Study the drawing (mm; zero at the part's minimum x, y, z) and answer. Round coordinates to 2 decimals unless told otherwise and drop trailing zeros. Write each loop counter-clockwise with the first axis right and the second up, starting at its lowest first coordinate (ties: lowest second). Pieces come first, ordered by that corner, then holes.
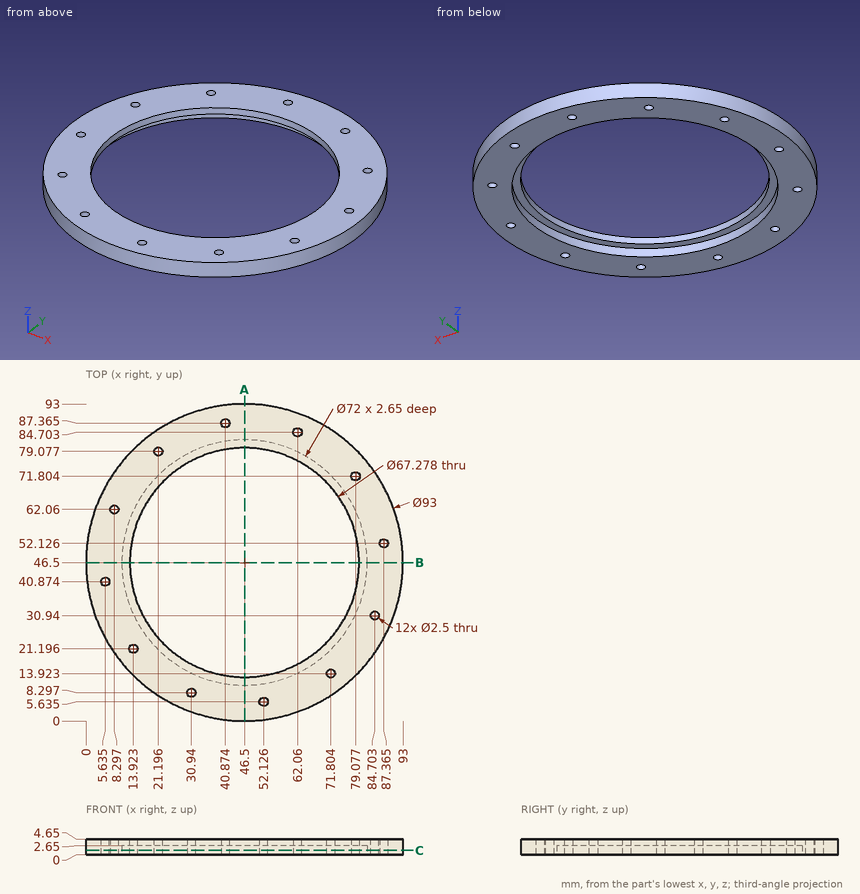
Q1. Given pin 1 (1.5 mm diameter, centred on y = 75.5, z = 1, fed in from -X) (1 decimal); pin 2 (3 mm diameter, centred on x = 62.06, y = 84.7, fed in from +Z); pin 3 (1.5 mm diameter, centred on x = 11, z = 3, fed in from +Y), each flat-ended and moving along its own axis, determine where each tip first touches the part or whether it passes through.
Q2. Find section C-C (z = 1.3). Count the separate pieces of the cut face and the enclosed holes in it, plus the area to 3 significant figures.
Q3. Find section A-A (x = 46.5). Determine the outline of the cut face in (y, z).
Q4. Find the intervals of material crossed by L1, parallel to Y at x = 40, z = 1.05 (1 decimal); L2, parallel to Y at x = 72, z = 3.75 (1 decimal); L3, parallel to Y at x = 45.5, z = 0.7, in increasing order.
Report:
1. pin 1: stops at x = 9.6
1. pin 2: stops at z = 4.65
1. pin 3: stops at y = 77.4
2. separate pieces: 1
2. enclosed holes: 13
2. area: 2,660 mm2
3. outline: (0, 0) - (10.5, 0) - (10.5, 2.65) - (12.86, 2.65) - (12.86, 4.65) - (0, 4.65) - close; (80.14, 2.65) - (82.5, 2.65) - (82.5, 0) - (93, 0) - (93, 4.65) - (80.14, 4.65) - close
4. L1: y = 0.5 to 11.1, 81.9 to 86.5, 88.3 to 92.5
4. L2: y = 7.6 to 12.7, 15.2 to 24.6, 68.4 to 85.4
4. L3: y = 0.01 to 10.51, 82.49 to 92.99
